Can you work these out from the model? Positions are in its coordinate system, mm. Give positions to 0.01 mm unless a question says otherwise; leave off trailing zeros. Loops run counter-clockwise (first coordinate to the right, second up) from the corner with the lowest first, then second, coordinate; pieces in that order, holes last. Notation, with made-up numbers: M 40.5,13.25 L 80.5,13.25 A15 ccw 80.5,22.25 Z; hole C -10,31.25 d1. An arc over 180 degrees is marked long. Put each result on its own line as item: value. Start each with the question number.
1) Please list where these lines run through material, in increasing order: line 1 along Y through (x, z) = (-32, 1.4); line 2 along Y through (x, z) = (-30.5, 0.8); line 3 along X through (y, z) = (-98.5, 1.4). Write a range as from..to.
2) If we mould it in two halves opening along Y, with no side actions, what happens to faces 1 (the flat face through (-49, -148, 2)), 2 (the cylindrical face through (-11.424, -84.002, 1.014))? For each: +Y half, -Y half, draft (parallel to the pull), parting line (faces both ways), or undercut.
3) Imagine slicing it at C-C (z = 1.1). Write out the boundary of the cut face in (x, y).
4) For P1, Ø1, axis at x = -47, y = -144, coming from the -Z side; P2, Ø1, axis at x = -21, z = 1, coming from the -Y side; P3, Ø1, axis at y = -288, z = 1.5, coming from the +X side, each with a flat end and sliding along its axis, tell me the tip position at first contact or that it passes through.
5) Imagine slicing it at B-B (y = -87). Write out the boundary of the cut face in (x, z), then the cut area to 3 significant figures.
6) Imagine slicing it at D-D (y = -118.5). Write out the boundary of the cut face in (x, z), then the cut area to 3 significant figures.
7) Imagine slicing it at A-A (x = -30.5). Write out the boundary of the cut face in (y, z).
from build123d import *

# Parameters (mm, degrees)
AUFSATZ_LINEAR_AUSTRAGEN1_DEPTH = 2
SKIZZE2_R                       = 20
SKIZZE2_R_2                     = 10
SCHNITT_LINEAR_AUSTRAGEN1_DEPTH = 10
DURCHGANGSLOCH_F_R_M61_D        = 6.6


with BuildPart() as part:
    # Skizze1 → Aufsatz-Linear austragen1 (new body)
    with BuildSketch(Plane.XY):
        Polygon((-4.0015, -24.009838693), (-27.0015, -24.009838693), (-27.0015, -0.009838693), (-93.0015, -0.009838693), (-93.0015, -300.009838693), (-27.0015, -300.009838693), (-27.0015, -276.009838693), (-4.0015, -276.009838693), align=None)
    extrude(amount=AUFSATZ_LINEAR_AUSTRAGEN1_DEPTH)

    # Skizze2 → Schnitt-Linear austragen1 (cut)
    with BuildSketch(Plane.XY.offset(2)):
        with Locations((-30.5, -90.009838693)):
            Circle(SKIZZE2_R)
        with Locations((-93.0015, -118.009838693)):
            Circle(SKIZZE2_R_2)
    extrude(amount=-SCHNITT_LINEAR_AUSTRAGEN1_DEPTH, mode=Mode.SUBTRACT)

    # Durchgangsloch für M61 (through all)
    with Locations(Plane.XY.offset(2)):
        with Locations((-19.0015, -39.009838693), (-19.0015, -261.009838693)):
            Hole(DURCHGANGSLOCH_F_R_M61_D / 2)


solid = part.part
Recorded:
1. line 1: -300.01..-109.95, -70.07..-0.01
1. line 2: -300.01..-110.01, -70.01..-0.01
1. line 3: -93..-48.61, -12.39..-4
2. face 1: draft
2. face 2: undercut
3. outline: M -93,-300.01 L -27,-300.01 L -27,-276.01 L -4,-276.01 L -4,-24.01 L -27,-24.01 L -27,-0.01 L -93,-0.01 L -93,-108.01 A10 cw -93,-128.01 Z; hole C -30.5,-90.01 d40; hole C -19,-261.01 d6.6; hole C -19,-39.01 d6.6
4. P1: z = 0
4. P2: y = -276.01
4. P3: x = -27
5. outline: M -93,0 L -50.27,0 L -50.27,2 L -93,2 Z; M -10.73,0 L -4,0 L -4,2 L -10.73,2 Z
5. area: 98.9 mm²
6. outline: M -83.01,0 L -4,0 L -4,2 L -83.01,2 Z
6. area: 158 mm²
7. outline: M -300.01,0 L -110.01,0 L -110.01,2 L -300.01,2 Z; M -70.01,0 L -0.01,0 L -0.01,2 L -70.01,2 Z
